Work out the finished part from the listing and answer in its coordinate system (mm). Face numbers are marked on the shaded views. A direction names the side the tool comes from. Coordinates: 2 decimals unless noted, no trailing zeros. Order: outer loops, then holes, each group sorted by start corner. A loop starts at its lowest first (then second) coordinate and runs counter-clockwise, first axis right, second up. Notation, with made-up numbers: (-7.5, 11.5) - (11.5, 11.5) arc R31 ccw to (11.5, 39.5) - close; hole circle Ø5 at (-9, -5). An arc over 180 degrees is marked (long way). Use CSV: the item, a comma, the result in double quotes. Start each with the question number.
Autodesk Inventor part; units mm, degrees
ref_plane "YZ Plane" through (0, 0, 0) normal (1, 0, 0) x (0, 1, 0)
ref_plane "XY Plane" through (0, 0, 0) normal (0, 0, 1) x (1, 0, 0)
sketch "Sketch1" plane through (0, 0, 0) normal (0, 0, 1) x (1, 0, 0)
  circle A0 centre (0, 0) radius 15
  circle A1 centre (150, 0) radius 25
  line L0 (-35, 45) -> (-35, -144.3782)
  circle A2 centre (20.0962, -75) radius 15
  line L1 (195, 45) -> (-35, 45)
  line L2 (195, -205) -> (0, -205)
  line L3 (195, -205) -> (195, 45)
  line L4 (0, -205) -> (-35, -144.3782)
  line L5 (0, -205) -> (70, -205) construction
  dimension "d0" = 230
  dimension "d1" = 120
extrude "Extrusion1" add sketch "Sketch1" along normal blind 210
fillet "Fillet1" radius 20 1 edges at (195, 45, 105)
fillet "Fillet2" radius 20 1 edges at (195, -205, 105)
fillet "Fillet3" radius 20 3 edges at (0, -205, 105) (-35, -144.3782, 105) (-35, 45, 105)
sketch "Sketch3" plane through (195, 25, 210) normal (1, 0, 0) x (0, 0, -1)
  line L0 (0, -210) -> (0, 0)
  line L1 (0, 20) -> (0, -230)
  line L2 (0, -230) -> (20, -230)
  line L3 (20, -230) -> (20, -180)
  line L4 (20, -180) -> (190, -180)
  line L5 (190, -180) -> (190, -230)
  line L6 (190, -230) -> (210, -230)
  line L7 (210, -230) -> (210, 20)
  line L8 (210, 20) -> (190, 20)
  line L9 (190, 20) -> (190, -150)
  line L10 (190, -150) -> (20, -150)
  line L11 (20, -150) -> (20, 20)
  line L12 (20, 20) -> (0, 20)
  point P0 (210, -25)
  dimension "d17" = 250
  dimension "d18" = 20
  dimension "d19" = 50
  dimension "d20" = 170
  dimension "d21" = 170
extrude "Extrusion3" cut sketch "Sketch3" against normal blind 230 keep common part
ref_plane "Work Plane1" through (175, -205, 10) normal (0, 1, 0) x (-1, 0, 0)
sketch "Sketch4" plane through (175, -205, 10) normal (0, 1, 0) x (-1, 0, 0)
  line L0 (210, -30) -> (220, -30)
  line L1 (220, -30) -> (220, 220)
  line L2 (220, 220) -> (-30, 220)
  line L3 (-30, 220) -> (-30, -30)
  line L4 (-30, -30) -> (210, -30)
  point P0 (175, -10)
  dimension "d25" = 10
  dimension "d26" = 250
  dimension "d27" = 250
  dimension "d28" = 250
extrude "Extrusion4" add sketch "Sketch4" against normal blind 20
properties part number "kepala 1 revisi"
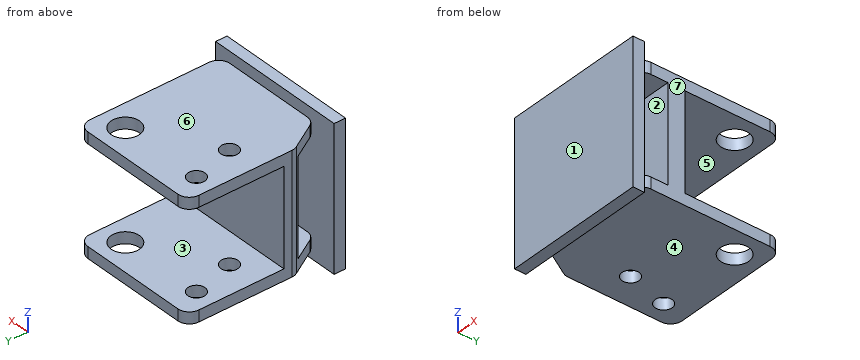
1) The part is cut by section D-D on y = 0. Determine the outline of the cut face in (x, z), plus the area to 3 significant figures.
2) The part is cut by section C-C on y = -75. Determine the outline of the cut face in (x, z), plus the area to 3 significant figures.
3) Flat-ended cylindrical pins translate along their axes: P1, Ø12, axis at x = 56.5, z = 168.5, coming from the +Y side; P2, Ø15, axis at x = 92.5, y = -184.5, coming from the +Z side; P3, Ø6, axis at x = -1, y = -196.5, coming from the -Z side. Find the tip coordinate at first contact, or state that the pin passes through.
4) For the marked faces 4, 5, 6 and 7, determine the directions among +Z, -Z, +X, -X, +Y, -Y from which every point of the face is accessible in a straight line to the end or side of a thin tool.
5) The part is cut by section B-B on z = 169. Determine the outline of the cut face in (x, y), plus the area to 3 significant figures.
6) Straight lines are drawn through the part: line 1 (X direction, y = 0, z = 196); line 2 (Z direction, x = -15, y = -101); line 3 (Y direction, x = 73.5, z = 75.5). For each, find the intervals that lie inside material, in ascending order. Write a range as [from, to].
7) For a pull along Y with two mould halves and no side action, classify the marked faces 1, 2 and 3 as +Y half, -Y half, draft (parallel to the pull), parting line (faces both ways), or undercut.
8) The part is cut by section A-A on x = 150. Determine the outline of the cut face in (y, z), plus the area to 3 significant figures.
Answer key:
1,outline,"(-35, 0) - (-15, 0) - (-15, 20) - (-35, 20) - close; (-35, 190) - (-15, 190) - (-15, 210) - (-35, 210) - close; (15, 0) - (125, 0) - (125, 20) - (15, 20) - close; (15, 190) - (125, 190) - (125, 210) - (15, 210) - close; (175, 0) - (195, 0) - (195, 20) - (175, 20) - close; (175, 190) - (195, 190) - (195, 210) - (175, 210) - close"
1,area,"6,000 mm^2"
2,outline,"(-35, 0) - (5.1, 0) - (5.1, 20) - (-35, 20) - close; (-35, 190) - (5.1, 190) - (5.1, 210) - (-35, 210) - close; (35.1, 0) - (195, 0) - (195, 20) - (35.1, 20) - close; (35.1, 190) - (195, 190) - (195, 210) - (35.1, 210) - close"
2,area,"8,000 mm^2"
3,P1,"y = -125"
3,P2,"z = 210"
3,P3,"z = 0"
4,face 4,"-Z, +X, -X, +Y"
4,face 5,"+X, -X, +Y"
4,face 6,"+Z, +X, -X, +Y"
4,face 7,"+Z, -Z, +X, +Y"
5,outline,"(-45, -225) - (205, -225) - (205, -205) - (-45, -205) - close; (-35, -139.02) arc R20 ccw to (-32.32, -149.02) - (-28.87, -155) - (195, -155) - (195, -125) - (-35, -125) - close"
5,area,"11,900 mm^2"
6,line 1,"[-35, -15], [15, 125], [175, 195]"
6,line 2,"[0, 20], [190, 210]"
6,line 3,"[-225, -205], [-155, -125]"
7,face 1,"-Y half"
7,face 2,"undercut"
7,face 3,"draft"
8,outline,"(-225, -20) - (-205, -20) - (-205, 0) - (-25, 0) - (-25, 20) - (-125, 20) - (-125, 190) - (-25, 190) - (-25, 210) - (-205, 210) - (-205, 230) - (-225, 230) - close; (25, 0) - (45, 0) - (45, 20) - (25, 20) - close; (25, 190) - (45, 190) - (45, 210) - (25, 210) - close; hole (-205, 20) - (-155, 20) - (-155, 190) - (-205, 190) - close"
8,area,"18,100 mm^2"
